from build123d import *

# Parameters (mm, degrees)
EXTRUDE_THIN1_DEPTH  = 15
SKETCH2_R            = 8.4
CUT_EXTRUDE1_DEPTH   = 69.574794932
FILLET1_R            = 12
FILLET1_OF_MIRROR1_R = 12
BOSS_EXTRUDE1_DEPTH  = 30


with BuildPart() as part:
    # Sketch1 → Extrude-Thin1 (new, symmetric)
    with BuildSketch(Plane.XY):
        Polygon((-63, 4.5), (-28, 4.5), (-28, 9.5), (-25.5, 9.5), (-25.5, 16), (-22, 16), (-22, 21.5), (-16.5, 21.5), (-16.5, 27.05), (0, 27.05), (0, 32.05), (-21.5, 32.05), (-21.5, 26.5), (-27, 26.5), (-27, 21), (-30.5, 21), (-30.5, 14.5), (-33, 14.5), (-33, 9.5), (-63, 9.5), align=None)
    extrude_thin1 = extrude(amount=EXTRUDE_THIN1_DEPTH, both=True)

    # Sketch2 → Cut-Extrude1 (cut, through all)
    with BuildSketch(Plane(origin=(0, 9.5, 0), x_dir=(1, 0, 0), z_dir=(0, 1, 0))):
        with Locations(Location((-45.8, 0, 0), (0, 0, 270))):
            Circle(SKETCH2_R)
    cut_extrude1 = extrude(amount=-CUT_EXTRUDE1_DEPTH, mode=Mode.SUBTRACT)

    # Fillet1
    fillet1_edges = [part.edges().sort_by_distance(p)[0] for p in [
        (-63, 7, -15),
        (-63, 7, 15),
    ]]
    fillet(fillet1_edges, radius=FILLET1_R)

    # Mirror1: Extrude-Thin1, Cut-Extrude1 across plane
    add(extrude_thin1.mirror(Plane(origin=(0, 32.05, 15), x_dir=(0, 0, 1), z_dir=(1, 0, 0))))
    add(cut_extrude1.mirror(Plane(origin=(0, 32.05, 15), x_dir=(0, 0, 1), z_dir=(1, 0, 0))), mode=Mode.SUBTRACT)

    # Fillet1 of Mirror1
    fillet1_of_mirror1_edges = [part.edges().sort_by_distance(p)[0] for p in [
        (63, 7, -15),
        (63, 7, 15),
    ]]
    fillet(fillet1_of_mirror1_edges, radius=FILLET1_OF_MIRROR1_R)

    # Sketch4 → Boss-Extrude1 (add)
    with BuildSketch(Plane(origin=(0, 0, -15), x_dir=(-1, 0, 0), z_dir=(0, 0, -1))):
        with BuildLine():
            Line((-34, 9.5), (-33, 9.5))
            Line((-33, 9.5), (-33, 14.5))
            Line((-33, 14.5), (-30.5, 14.5))
            Line((-30.5, 14.5), (-30.5, 21))
            Line((-30.5, 21), (-27, 21))
            Line((-27, 21), (-27, 26.5))
            Line((-27, 26.5), (-21.5, 26.5))
            Line((-21.5, 26.5), (-21.5, 32.05))
            ThreePointArc((-21.5, 32.05), (-30.55647166, 22.330693825), (-34, 9.5))
        make_face()
    boss_extrude1 = extrude(amount=-BOSS_EXTRUDE1_DEPTH)

    # Mirror2: Boss-Extrude1 across plane
    add(boss_extrude1.mirror(Plane(origin=(0, 0, 0), x_dir=(0, 0, 1), z_dir=(1, 0, 0))))


solid = part.part
Source: CAD feature listing. Evaluate the final solid. Frame: model axes, mm. A direction names the side the tool comes from. Round coordinates to 2 decimals unless told otherwise and drop trailing zeros. Loops run counter-clockwise (first coordinate to the right, second up) from the corner with the lowest first, then second, coordinate; pieces in that order, holes last. Notation, with made-up numbers: M 20,64 L 45,64 A29 ccw 45,92 Z; hole C 45.5,49 d5. An arc over 180 degrees is marked long. Answer as CSV lines item,"result".
Q1. Cut plane A-A (y = 7.25). Return the cut outline in (x, z).
Verdict:
outline,"M -63,-3 A12 ccw -51,-15 L -28,-15 L -28,15 L -51,15 A12 ccw -63,3 Z; M 28,-15 L 51,-15 A12 ccw 63,-3 L 63,3 A12 ccw 51,15 L 28,15 Z; hole C -45.8,0 d16.8; hole C 45.8,0 d16.8"
Q2. Cut plane C-C (x = 45.8). Return the cut outline in (y, z), plus the area to 3 significant figures.
Verdict:
outline,"M 4.5,-15 L 9.5,-15 L 9.5,-8.4 L 4.5,-8.4 Z; M 4.5,8.4 L 9.5,8.4 L 9.5,15 L 4.5,15 Z"
area,"66.0 mm^2"
Q3. Pull-direction query (Z, two-part tool) for faces 1 (the face through (54, 7.04, -1.82)), 2 (the face through (0, 30, 15)), 3 (the face through (-38, 4.5, 4)); classes: +Z half, -Z half, draft (parallel to the pull), parting line (faces both ways), or undercut.
Verdict:
face 1,"undercut"
face 2,"+Z half"
face 3,"draft"
Q4. Reachability of faces 4 (the face through (55, 9.5, 0)), 5 (the face through (28, 7, 0)), 6 (the face through (-59.39, 6.96, -11.58)) from +Z, -Z, +X, -X, +Y, -Y: full face, straight path, thin tool, end or side. Return the list, or none.
Verdict:
face 4,"+Z, -Z, +X, +Y"
face 5,"+Z, -Z, -Y"
face 6,"-Z, -X, +Y, -Y"
Q5. Line query: line 1 along X through (y, z) = (8.2, 0); line 2 along X through (y, z) = (10.25, 11.5); line 3 along Z through (x, y) = (45.8, 5.5). Output: solid intervals per line, ascending.
Verdict:
line 1,"x = -63 to -54.2, -37.4 to -28, 28 to 37.4, 54.2 to 63"
line 2,"x = -33.98 to -25.5, 25.5 to 33.98"
line 3,"z = -15 to -8.4, 8.4 to 15"
Q6. Cut plane D-D (y = 14.75). Return the cut outline in (x, z).
Verdict:
outline,"M -33.4,-15 L -25.5,-15 L -25.5,15 L -33.4,15 Z; M 25.5,-15 L 33.4,-15 L 33.4,15 L 25.5,15 Z"
Q7. Cut plane B-B (z = 0). Count the separate pieces of the cut face and the enclosed holes in it, plus the area to 3 significant figures.
Verdict:
separate pieces,"3"
enclosed holes,"0"
area,"789 mm^2"
Q8. Contact query for flat-ended pins moving along their axis: pin 1 (10 mm diameter, centred on y = 12, z = -1.5, fed in from +X); pin 2 (1.5 mm diameter, centred on y = 15.5, z = 0.5, fed in from +X); pin 3 (2 mm diameter, centred on x = 26.5, z = 6, fed in from -Y); pin 4 (1.8 mm diameter, centred on x = 23.5, z = -4.5, fed in from -Y). Output: stop coordinate, or through.
Verdict:
pin 1,"stops at x = 63"
pin 2,"stops at x = 33.4"
pin 3,"stops at y = 9.5"
pin 4,"stops at y = 16"
